Read the model definition and answer for the solid it produces. Units are mm, in the model's axes. A direction names the side the tool comes from. Coordinates: 2 decimals unless noted, no trailing zeros. Loops run counter-clockwise (first coordinate to the right, second up) from the corner with the lowest first, then second, coordinate; pieces in that order, holes last. Notation, with made-up numbers: (35, 56.25) -> (59, 56.25) arc R5 cw to (59, 65.25) -> close; hole circle Ø7 at (-28, 70.25). An arc over 180 degrees is marked (long way). Answer as a JSON object with one key per item and string values. Group by question number.
1) Section B-B, the plane y = 7 is taken. Give the vertices of the cut face in (x, z).
2) Section A-A, the plane z = 36 is taken. Give the vertices of the cut face in (x, y).
3) Section D-D, the plane z = 22.5 is taken. Give the vertices of the cut face in (x, y), plus the area to 3 significant figures.
4) Determine the mould class of faces 3 (the face through (0, 13, 22)), 4 (the face through (22, 15, 44.45)), 5 (the face through (21.24, 6.26, 40.62)), 6 (the face through (15.054, 12.522, 17.403)) for opening direction X: released by +X, released by -X, zero draft, split by the parting line, or undercut.
5) Which of the six approach directions +Z, -Z, +X, -X, +Y, -Y give full straight-line access (tool end or side, diameter ignored) to faces 1 (the face through (42, 12.7, 27)), 2 (the face through (12, 0, 18))?
6) Flat-ended cylindrical pins translate along their axes: P1, Ø12, axis at x = 51, z = 33, coming from the -Y side; P2, Ø1.5, axis at y = 5.5, z = 23.5, coming from the +X side. Find the tip coordinate at first contact, or state that the pin passes through.
7) Section C-C, the plane x = 42.5 is taken. Give the vertices of the cut face in (y, z).
8) Consider probe 1 along Z at (x, y) = (25, 19.75); probe 2 along Y at (x, z) = (25, 41.5); probe 3 along Z at (x, y) = (26, 22.25). Determine where each line is inside the solid, lowest interval first. Write a range as [from, to].
from build123d import *

# Parameters (mm, degrees)
F0_W     = 57.15
F0_H     = 44.45
F1_DEPTH = 25.4
F2_W     = 12.7
F2_H     = 44.45
F3_DEPTH = 12.7
F5_DEPTH = 12.7
F6_R     = 12.012115
F7_DEPTH = 25.4


with BuildPart() as f1:
    # F0 (on Front) → F1 (new body)
    with BuildSketch(Plane.XZ):
        with Locations((28.575, 22.225)):
            Rectangle(F0_W, F0_H)
    extrude(amount=-F1_DEPTH)

    # F2 (on Front) → F3 (cut)
    with BuildSketch(Plane.XZ):
        with Locations((50.8, 22.225)):
            Rectangle(F2_W, F2_H)
    extrude(amount=-F3_DEPTH, mode=Mode.SUBTRACT)

    # F4 (on Front) → F5 (cut)
    with BuildSketch(Plane.XZ):
        Polygon((19.05, 44.45), (44.45, 0), (44.45, 44.45), align=None)
    extrude(amount=-F5_DEPTH, mode=Mode.SUBTRACT)

    # F6 (on Front) → F7 (cut)
    with BuildSketch(Plane.XZ):
        with Locations((24.58664, 24.712115)):
            Circle(F6_R)
    extrude(amount=-F7_DEPTH, mode=Mode.SUBTRACT)


solid = f1.part
Determined:
{
 "1": {"outline": "(0, 0) -> (44.45, 0) -> (34.34, 17.7) arc R12.01 cw (long way) to (23.49, 36.67) -> (19.05, 44.45) -> (0, 44.45) -> close"},
 "2": {"outline": "(0, 0) -> (20.48, 0) -> (20.48, 25.4) -> (0, 25.4) -> close; (28.69, 12.7) -> (57.15, 12.7) -> (57.15, 25.4) -> (28.69, 25.4) -> close"},
 "3": {"outline": "(0, 0) -> (12.78, 0) -> (12.78, 25.4) -> (0, 25.4) -> close; (36.39, 12.7) -> (57.15, 12.7) -> (57.15, 25.4) -> (36.39, 25.4) -> close", "area": "588 mm²"},
 "4": {"face 3": "released by -X", "face 4": "zero draft", "face 5": "released by +X", "face 6": "undercut"},
 "5": {"face 1": "+Z, +X, -Y", "face 2": "+Z, -Z, +X, -X, -Y"},
 "6": {"P1": "y = 12.7", "P2": "x = 12.74"},
 "7": {"outline": "(0, 0) -> (25.4, 0) -> (25.4, 44.45) -> (12.7, 44.45) -> (12.7, 3.41) -> (0, 3.41) -> close"},
 "8": {"probe 1": "[0, 12.71], [36.72, 44.45]", "probe 2": "[12.7, 25.4]", "probe 3": "[0, 12.78], [36.64, 44.45]"}
}
